Source: CAD feature listing. Evaluate the final solid. Frame: model axes, mm. A direction names the side the tool comes from. Give positions to 0.01 mm unless a question says otherwise; leave off trailing zeros. Order: outer loops, then holes, each group sorted by start corner. A loop starts at its lowest first (then second) coordinate and runs counter-clockwise, first axis right, second up. Notation, with made-up numbers: M -16.75,-28.75 L 30.25,-28.75 A22 ccw 30.25,-8.75 Z; hole C 41.25,-38.5 d10. An arc over 180 degrees is marked long. Answer as a JSON object with one key per item and string values. Group by question number.
1. Section query C-C (y = -473.5). Output: boundary loops of the cut face in (x, z), plus the area to 3 significant figures.
2. Pull-direction query (Z, two-part tool) for faces 4 (the flat face through (-499, -36, -434)), 5 (the flat face through (-499.507, 420.062, 239.425)), 6 (the cylindrical face through (-499.507, -498.192, -42.478)); classes: +Z half, -Z half, draft (parallel to the pull), parting line (faces both ways), or undercut.
3. Section query A-A (x = -499.55). Output: boundary loops of the cut face in (y, z).
4. Material intervals for L1, parallel to Y at x = -499.9, z = -715; L2, parallel to Y at x = -499.9, z = 669; L3, parallel to Z at x = -499.85, y = 312.5, sorted ascending. Write a range as [from, to].
5. Pin query (flat end, axial travel): P1, Ø0.5, axis at x = -499.5, z = -994, coming from the -Y side. Return the tip coordinate at first contact, or that it passes through.
6. Section query D-D (z = 890). Output: boundary loops of the cut face in (x, y).
7. Set-up query: faces 1 (the flat face through (-500, -36, -434)), 2 (the flat face through (-499.51, 492, -417.07)), 3 (the flat face through (-499.507, -542.976, 391.604)). Return all of +Z, -Z, +X, -X, +Y, -Y with unobstructed straight access to the full face (end or side cutting, diameter ignored); none if empty.
8. Section query B-B (y = 423.5). Output: boundary loops of the cut face in (x, z).
from build123d import *

# Parameters (mm, degrees)
PAD_DEPTH = 1


with BuildPart() as part:
    # Sketch → Pad (new body)
    with BuildSketch(Plane.YZ.offset(-500)):
        with BuildLine():
            ThreePointArc((-434.556983, 247.305941), (-497.810755, -46.738128), (-380.9308, -323.869921))
            Line((-380.9308, -323.869921), (-600, -507.690796))
            Line((-600, -507.690796), (-600, -1400))
            Line((-600, -1400), (600, -1400))
            Line((600, -1400), (600, -507.690796))
            Line((600, -507.690796), (380.9308, -323.869921))
            ThreePointArc((380.9308, -323.869921), (424.161816, -264.739029), (458.28967, -199.926432))
            Line((458.28967, 180.073568), (458.28967, -199.926432))
            Line((382.889757, 297.136749), (458.28967, 180.073568))
            Line((312.889757, 297.136749), (382.889757, 297.136749))
            Line((312.889757, 390), (312.889757, 297.136749))
            Line((199.509467, 390), (312.889757, 390))
            Line((199.509467, 458.471343), (199.509467, 390))
            Line((3.8e-05, 458.471343), (199.509467, 458.471343))
            Line((3.8e-05, 500), (3.8e-05, 458.471343))
            Line((-152.007187, 500), (3.8e-05, 500))
            Line((-152.007187, 1040), (-152.007187, 500))
            Line((-654.474365, 1040), (-152.007187, 1040))
            Line((-654.474365, 1040), (-654.474365, 540))
            Line((-434.556983, 247.305941), (-654.474365, 540))
        make_face()
    extrude(amount=PAD_DEPTH)


solid = part.part
Answer sheet:
{
 "1": {"outline": "M -500,-1400 L -499,-1400 L -499,-401.54 L -500,-401.54 Z; M -500,-160.62 L -499,-160.62 L -499,160.62 L -500,160.62 Z; M -500,299.14 L -499,299.14 L -499,1040 L -500,1040 Z", "area": "2,060 mm^2"},
 "2": {"face 4": "draft", "face 5": "+Z half", "face 6": "undercut"},
 "3": {"outline": "M -654.47,540 L -434.56,247.31 A500 ccw -380.93,-323.87 L -600,-507.69 L -600,-1400 L 600,-1400 L 600,-507.69 L 380.93,-323.87 A500 ccw 458.29,-199.93 L 458.29,180.07 L 382.89,297.14 L 312.89,297.14 L 312.89,390 L 199.51,390 L 199.51,458.47 L 0,458.47 L 0,500 L -152.01,500 L -152.01,1040 L -654.47,1040 Z"},
 "4": {"L1": "[-600, 600]", "L2": "[-654.47, -152.01]", "L3": "[-1400, 390]"},
 "5": {"P1": "y = -600"},
 "6": {"outline": "M -500,-654.47 L -499,-654.47 L -499,-152.01 L -500,-152.01 Z"},
 "7": {"face 1": "+Z, -Z, -X, +Y, -Y", "face 2": "+X, -X, +Y", "face 3": "+X, -X, -Y"},
 "8": {"outline": "M -500,-1400 L -499,-1400 L -499,-359.59 L -500,-359.59 Z; M -500,-265.8 L -499,-265.8 L -499,234.09 L -500,234.09 Z"}
}
